```python
from build123d import *

# Parameters (mm, degrees)
BOSS_EXTRUDE1_DEPTH = 75
SKETCH3_W           = 30
SKETCH3_H           = 35
CUT_EXTRUDE1_DEPTH  = 75
BOSS_EXTRUDE2_DEPTH = 40
BOSS_EXTRUDE3_DEPTH = 26
SKETCH6_R           = 10
CUT_EXTRUDE2_DEPTH  = 97.492272876
BOSS_EXTRUDE4_DEPTH = 37
CUT_EXTRUDE3_DEPTH  = 35
SKETCH9_R           = 5
CUT_EXTRUDE4_DEPTH  = 35


with BuildPart() as part:
    # Sketch2 → Boss-Extrude1 (new body)
    with BuildSketch(Plane(origin=(0, 0, 0), x_dir=(0, 0, -1), z_dir=(1, 0, 0))):
        Polygon((-68.973908168, 0), (-68.973908168, 15), (-3.973908168, 15), (-3.973908168, 25), (31.026091832, 25), (31.026091832, 0), align=None)
    extrude(amount=-BOSS_EXTRUDE1_DEPTH)

    # Sketch3 → Cut-Extrude1 (cut)
    with BuildSketch(Plane(origin=(0, 15, 0), x_dir=(1, 0, 0), z_dir=(0, 1, 0))):
        with Locations((-60, -51.473908168)):
            Rectangle(SKETCH3_W, SKETCH3_H)
    extrude(amount=-CUT_EXTRUDE1_DEPTH, mode=Mode.SUBTRACT)

    # Sketch4 → Boss-Extrude2 (add)
    with BuildSketch(Plane.ZY.offset(75)):
        Polygon((3.973908168, 25), (21.294416244, 15), (3.973908168, 15), align=None)
    extrude(amount=-BOSS_EXTRUDE2_DEPTH)

    # Sketch5 → Boss-Extrude3 (add)
    with BuildSketch(Plane(origin=(0, 20.470752713, 11.818794589), x_dir=(1, 0, 0), z_dir=(0, 0.866025403784438, 0.5000000000000012))):
        with BuildLine():
            Line((-75, 9.058494574), (-35, 9.058494574))
            ThreePointArc((-35, 9.058494574), (-55, 29.058494574), (-75, 9.058494574))
        make_face()
    extrude(amount=-BOSS_EXTRUDE3_DEPTH)

    # Sketch6 → Cut-Extrude2 (cut, through all)
    with BuildSketch(Plane(origin=(0, 20.470752713, 11.818794589), x_dir=(1, 0, 0), z_dir=(0, 0.866025403784438, 0.5000000000000012))):
        with Locations(Location((-55, 9.058494574, 0), (0, 0, 270))):
            Circle(SKETCH6_R)
    extrude(amount=-CUT_EXTRUDE2_DEPTH, mode=Mode.SUBTRACT)

    # Sketch8 → Boss-Extrude4 (add)
    with BuildSketch(Plane(origin=(0, 0, 0), x_dir=(0, 0, -1), z_dir=(1, 0, 0))):
        with BuildLine():
            Line((-21.294416244, 15), (-14.754270695, 15))
            ThreePointArc((-14.754270695, 15), (-8.612251296, 19.189491233), (-3.973908168, 25))
            Line((-3.973908168, 25), (-21.294416244, 15))
        make_face()
        with BuildLine():
            ThreePointArc((-3.973908168, 25), (-8.612251296, 19.189491233), (-14.754270695, 15))
            Line((-14.754270695, 15), (-3.973908168, 15))
            Line((-3.973908168, 15), (-3.973908168, 25))
        make_face()
    extrude(amount=-BOSS_EXTRUDE4_DEPTH)

    # Sketch8_3 → Cut-Extrude3 (cut)
    with BuildSketch(Plane(origin=(0, 0, 0), x_dir=(0, 0, -1), z_dir=(1, 0, 0))):
        with BuildLine():
            Line((-21.294416244, 15), (-14.754270695, 15))
            ThreePointArc((-14.754270695, 15), (-8.612251296, 19.189491233), (-3.973908168, 25))
            Line((-3.973908168, 25), (-21.294416244, 15))
        make_face()
        with BuildLine():
            ThreePointArc((-36.473908168, 15), (-25.614089432, 12.518089107), (-14.754270695, 15))
            Line((-14.754270695, 15), (-21.294416244, 15))
            Line((-21.294416244, 15), (-36.473908168, 15))
        make_face()
    extrude(amount=-CUT_EXTRUDE3_DEPTH, mode=Mode.SUBTRACT)

    # Sketch9 → Cut-Extrude4 (cut)
    with BuildSketch(Plane(origin=(0, 25, 0), x_dir=(1, 0, 0), z_dir=(0, 1, 0))):
        with Locations(Location((-15, 16.026091832, 0), (0, 0, 270))):
            Circle(SKETCH9_R)
        with Locations(Location((-15, -58.973908168, 0), (0, 0, 270))):
            Circle(SKETCH9_R)
    extrude(amount=-CUT_EXTRUDE4_DEPTH, mode=Mode.SUBTRACT)


solid = part.part
```
Work out the finished part from the listing and answer in its coordinate system (mm). A direction names the side the tool comes from. Round coordinates to 2 decimals unless told otherwise and drop trailing zeros. Write each loop counter-clockwise with the first axis right and the second up, starting at its lowest first coordinate (ties: lowest second). Pieces come first, ordered by that corner, then holes. Notation, with made-up numbers: (70.25, 41) - (129.25, 41) arc R35 ccw to (129.25, 77) - close; hole circle Ø2 at (0, 46.25). An arc over 180 degrees is marked (long way). Return JSON: item names as keys, results as strings. Group by question number.
Q1. The part is cut by section A-A on x = -15. Write down the section's boundary in (y, z), then the cut area to 3 significant figures.
Q2. For faces 4 (the flat face through (-35, 16, 18)), 5 (the flat face through (-29, 15, 45)), 6 (the flat face through (-45, 8, 52)), determine the directions among +Z, -Z, +X, -X, +Y, -Y from which every point of the face is accessible in a straight line to the end or side of a thin tool.
Q3. The part is cut by section D-D on x = -49. Write down the section's boundary in (y, z).
Q4. The part is cut by section B-B on x = -33. Write down the section's boundary in (y, z), then the cut area to 3 significant figures.
Q5. Each of these flat-tipped pins is pushed along its axis until it touches: pin 1 Ø7.5 at (y, z) = (6.5, 52.5) entering from -X; pin 2 Ø5 at (x, y) = (-41, 22.5) entering from +Z; pin 3 Ø10 at (y, z) = (19.5, 27) entering from +X; pin 4 Ø8 at (x, z) = (-15, 58.97) entering from -Y. Where does it stop, or does it pass through?
Q6. The part is cut by section C-C on z = 62. Write down the section's boundary in (x, y), then the cut area to 3 significant figures.
Q7. Find the intervals of material crossed by L1, parallel to Y at x = -36, z = -25.5; L2, parallel to Y at x = -8.5, z = 41; L3, parallel to X at y = 16.5, z = 6, in increasing order.
Q8. The mould has two halves that part along Z. Classify faces 1 (the flat face through (-60, 8, 33.974)), 2 (the cylindrical face through (-18.042, 7.605, 55.006)), 3 (the flat face through (-37, 13, -31.026)): released by +Z, released by -Z, zero draft, split by the parting line, or undercut.
Solved:
{
 "1": {"outline": "(0, -31.03) - (25, -31.03) - (25, -21.03) - (0, -21.03) - close; (0, -11.03) - (25, -11.03) - (25, 3.97) arc R25 cw to (15, 36.47) - (15, 53.97) - (0, 53.97) - close; (0, 63.97) - (15, 63.97) - (15, 68.97) - (0, 68.97) - close", "area": "1,460 mm²"},
 "2": {"face 4": "+X, +Y", "face 5": "+Z, +X, -X, +Y", "face 6": "+Z, -X, +Y, -Y"},
 "3": {"outline": "(0, -31.03) - (25, -31.03) - (25, -18.06) - (34.54, -12.55) - (29, -2.95) - (0, -19.7) - close; (0, -1.22) - (21, 10.9) - (15, 21.29) - (15, 33.97) - (0, 33.97) - close"},
 "4": {"outline": "(0, -31.03) - (25, -31.03) - (25, 3.97) arc R25 cw to (15, 36.47) - (15, 68.97) - (0, 68.97) - close", "area": "1,860 mm²"},
 "5": {"pin 1": "x = -45", "pin 2": "z = 12.63", "pin 3": "x = -35", "pin 4": "through"},
 "6": {"outline": "(-45, 0) - (-18.98, 0) - (-18.98, 15) - (-45, 15) - close; (-11.02, 0) - (0, 0) - (0, 15) - (-11.02, 15) - close", "area": "556 mm²"},
 "7": {"L1": "0 to 25", "L2": "0 to 15", "L3": "-75 to -63, -47 to 0"},
 "8": {"face 1": "released by +Z", "face 2": "undercut", "face 3": "released by -Z"}
}
